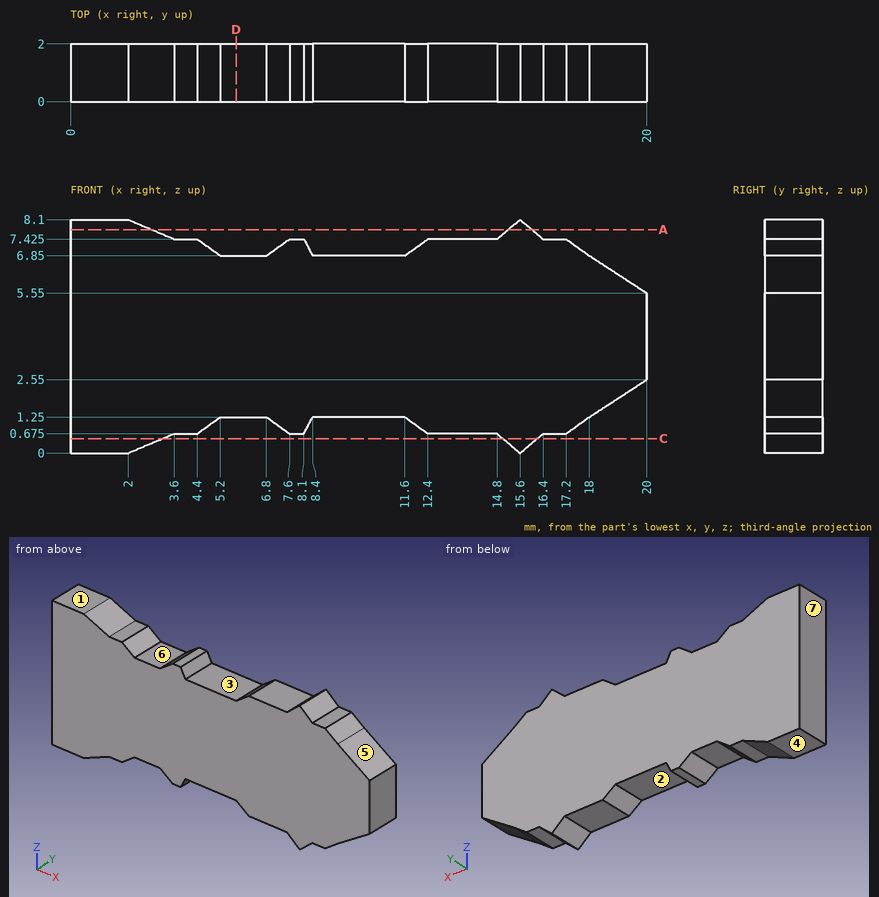
For this review, use the dimensioned drawing (mm, ordinates from the lowest corner) and the shaded views. A direction names the side the tool comes from. Coordinates: 2 decimals unless noted, no trailing zeros. Write each loop counter-clockwise with the first axis right and the second up, starting at its lowest first coordinate (ties: lowest second). Pieces come first, ordered by that corner, then holes. Notation, with made-up numbers: (20, 58.5) - (52, 58.5) arc R11 cw to (52, 79.5) - close; hole circle Ø9 at (31.25, 48.5). An arc over 180 degrees is marked (long way). Answer as a JSON object with one key per item and string values. Group by question number.
1. Clearance check with flat-ended pins moving along their axes: pin 1 Ø0.6 at (x, y) = (14, 1) entering from -Z (3 decimals); pin 2 Ø0.9 at (x, y) = (4, 1.5) entering from +Z; pin 3 Ø1 at (x, z) = (8.5, 1) entering from +Y. State where each tip first meets the part, or that it passes through.
2. Machinability: for the marked faces 1, 2 and 3, which of the approach directions +Z, -Z, +X, -X, +Y, -Y give a long, thin tool a straight path to every point of the face, cutting with its end or side? Answer none if there is none.
3. Add section A-A (z = 7.75). Give the boundary of the cut face in (x, y), plus the area to 3 significant figures.
4. Add section D-D (x = 5.75). Give the boundary of the cut face in (y, z), plus the area to 3 significant figures.
5. To check wall thickness, follow probe 1 along X at (y, z) = (1.05, 7.5); probe 2 along Z at (x, y) = (11.25, 0.8); probe 3 along Z at (x, y) = (14.5, 1.8) (3 decimals). State the ranges of each line that lie inside material, in increasing order.
6. Mouldability with a two-part tool opening along X and no side actions: class the marked faces 4, 5, 6 and 7 as pulls with the +X half, pulls with the -X half, needs draft (parallel to the pull), parting line crosses it, or undercut.
7. Add section C-C (z = 0.5). Give the boundary of the cut face in (x, y).
Findings:
{
 "1": {"pin 1": "z = 0.675", "pin 2": "z = 7.45", "pin 3": "y = 2"},
 "2": {"face 1": "+Z, +X, -X, +Y, -Y", "face 2": "-Z, +Y, -Y", "face 3": "+Z, +Y, -Y"},
 "3": {"outline": "(0, 0) - (2.83, 0) - (2.83, 2) - (0, 2) - close; (15.19, 0) - (16.01, 0) - (16.01, 2) - (15.19, 2) - close", "area": "7.32 mm²"},
 "4": {"outline": "(0, 1.25) - (2, 1.25) - (2, 6.85) - (0, 6.85) - close", "area": "11.2 mm²"},
 "5": {"probe 1": "0 to 3.42, 14.89 to 16.31", "probe 2": "1.25 to 6.85", "probe 3": "0.675 to 7.425"},
 "6": {"face 4": "needs draft", "face 5": "pulls with the +X half", "face 6": "undercut", "face 7": "pulls with the -X half"},
 "7": {"outline": "(0, 0) - (3.19, 0) - (3.19, 2) - (0, 2) - close; (15.01, 0) - (16.19, 0) - (16.19, 2) - (15.01, 2) - close"}
}
